from build123d import *

# Parameters (mm, degrees)
F0_W         = 27.2
F0_H         = 4.4
F0_W_2       = 4.4
F0_H_2       = 33.7
F1_DEPTH     = 3
F2_R         = 2.99999
F3_DEPTH     = 2
F4_W         = 4.4
F4_H         = 4.4
F5_DEPTH     = 1
F6_T1_DEPTH  = 16
F6_T4_ANGLE  = 90
F6_T6_ANGLE  = 90
F6_T8_ANGLE  = 90
F6_T10_ANGLE = 90


# Not quite as in the source:
# - a fillet or chamfer that OpenCascade refuses, or shapes differently, is made with other operations: its cross-section is extruded or revolved along the edge and cut away or added
# - a fillet or chamfer is up to 0.001 mm smaller than in the source, because OpenCascade refuses the exact size


with BuildPart() as f1:
    # F0 (on Top) → F1 (new body)
    with BuildSketch(Plane.XY):
        with Locations((0.1669520199, 19.5440534235)):
            Rectangle(F0_W, F0_H)
        with Locations((-15.6330479801, 0.4940534235)):
            Rectangle(F0_W_2, F0_H_2)
        with Locations((-15.6330479801, 19.5440534235)):
            Rectangle(F0_W_2, F0_H)
        with Locations((-15.6330479801, -18.5559465765)):
            Rectangle(F0_W_2, F0_H)
        with Locations((0.1669520199, -18.5559465765)):
            Rectangle(F0_W, F0_H)
        with Locations((15.9669520199, -18.5559465765)):
            Rectangle(F0_W_2, F0_H)
        with Locations((15.9669520199, 0.4940534235)):
            Rectangle(F0_W_2, F0_H_2)
        with Locations((15.9669520199, 19.5440534235)):
            Rectangle(F0_W_2, F0_H)
    extrude(amount=F1_DEPTH)

    # F2 (radius 3 in the source; OpenCascade refuses exactly that, so slightly less here)
    f2_edges = [f1.edges().sort_by_distance(p)[0] for p in [
        (18.166952, 0.494053, 3),
        (0.166952, 21.744053, 3),
        (-17.833048, 0.494053, 3),
        (0.166952, -20.755947, 3),
    ]]
    fillet(f2_edges, radius=F2_R)

    # F0 (on Top) → F3 (join)
    with BuildSketch(Plane.XY):
        with Locations((-15.6330479801, -18.5559465765)):
            Rectangle(F0_W_2, F0_H)
        with Locations((15.9669520199, -18.5559465765)):
            Rectangle(F0_W_2, F0_H)
        with Locations((15.9669520199, 19.5440534235)):
            Rectangle(F0_W_2, F0_H)
        with Locations((-15.6330479801, 19.5440534235)):
            Rectangle(F0_W_2, F0_H)
    extrude(amount=-F3_DEPTH)

    # F4 (on face) → F5 (join)
    with BuildSketch(Plane(origin=(0, 0, -2), x_dir=(1, 0, 0), z_dir=(0, 0, -1))):
        Polygon((-13.4330479801, -21.7440534235), (18.1669520199, -21.7440534235), (18.1669520199, 20.7559465765), (-17.8330479801, 20.7559465765), (-17.8330479801, -17.3440534235), (-13.4330479801, -17.3440534235), align=None)
        with Locations((-15.6330479801, -19.5440534235)):
            Rectangle(F4_W, F4_H)
    extrude(amount=F5_DEPTH)

    # F6: fillet of radius 4 on 4 edges, made by hand

    # F6_s2 → F6_t1 (cut)
    with BuildSketch(Plane.XY.offset(-13)):
        with BuildLine():
            ThreePointArc((18.1669520199, 17.7440534235), (16.9953791447, 20.5724805482), (14.1669520199, 21.7440534235))
            Line((14.1669520199, 21.7440534235), (18.1669520199, 21.7440534235))
            Line((18.1669520199, 21.7440534235), (18.1669520199, 17.7440534235))
        make_face()
        with BuildLine():
            ThreePointArc((18.1669520199, -16.7559465765), (16.9953791447, -19.5843737013), (14.1669520199, -20.7559465765))
            Line((14.1669520199, -20.7559465765), (18.1669520199, -20.7559465765))
            Line((18.1669520199, -20.7559465765), (18.1669520199, -16.7559465765))
        make_face()
        with BuildLine():
            ThreePointArc((-17.8330479801, -16.7559465765), (-16.6614751048, -19.5843737013), (-13.8330479801, -20.7559465765))
            Line((-13.8330479801, -20.7559465765), (-17.8330479801, -20.7559465765))
            Line((-17.8330479801, -20.7559465765), (-17.8330479801, -16.7559465765))
        make_face()
        with BuildLine():
            ThreePointArc((-17.8330479801, 17.7440534235), (-16.6614751048, 20.5724805482), (-13.8330479801, 21.7440534235))
            Line((-13.8330479801, 21.7440534235), (-17.8330479801, 21.7440534235))
            Line((-17.8330479801, 21.7440534235), (-17.8330479801, 17.7440534235))
        make_face()
    extrude(amount=F6_T1_DEPTH, mode=Mode.SUBTRACT)

    # F6_s3 → F6_t4 (revolve, cut)
    with BuildSketch(Plane.YZ.offset(-13.8330479801)):
        with BuildLine():
            ThreePointArc((18.7440634235, 3), (20.8653766959, 2.1213232725), (21.7440534235, 1e-05))
            Line((21.7440534235, 1e-05), (21.7440534235, 3))
            Line((21.7440534235, 3), (18.7440634235, 3))
        make_face()
    revolve(axis=Axis((-13.8330479801, 17.7440534235, 3), (0, 0, 1)), revolution_arc=F6_T4_ANGLE, mode=Mode.SUBTRACT)

    # F6_s5 → F6_t6 (revolve, cut)
    with BuildSketch(Plane.XZ.offset(16.7559465765)):
        with BuildLine():
            ThreePointArc((-14.8330579801, 3), (-16.9543712526, 2.1213232725), (-17.8330479801, 1e-05))
            Line((-17.8330479801, 1e-05), (-17.8330479801, 3))
            Line((-17.8330479801, 3), (-14.8330579801, 3))
        make_face()
    revolve(axis=Axis((-13.8330479801, -16.7559465765, 3), (0, 0, 1)), revolution_arc=F6_T6_ANGLE, mode=Mode.SUBTRACT)

    # F6_s7 → F6_t8 (revolve, cut)
    with BuildSketch(Plane.YZ.offset(14.1669520199)):
        with BuildLine():
            ThreePointArc((-17.7559565765, 3), (-19.877269849, 2.1213232725), (-20.7559465765, 1e-05))
            Line((-20.7559465765, 1e-05), (-20.7559465765, 3))
            Line((-20.7559465765, 3), (-17.7559565765, 3))
        make_face()
    revolve(axis=Axis((14.1669520199, -16.7559465765, 3), (0, 0, 1)), revolution_arc=F6_T8_ANGLE, mode=Mode.SUBTRACT)

    # F6_s9 → F6_t10 (revolve, cut)
    with BuildSketch(Plane.XZ.offset(-17.7440534235)):
        with BuildLine():
            ThreePointArc((15.1669620199, 3), (17.2882752924, 2.1213232725), (18.1669520199, 1e-05))
            Line((18.1669520199, 1e-05), (18.1669520199, 3))
            Line((18.1669520199, 3), (15.1669620199, 3))
        make_face()
    revolve(axis=Axis((14.1669520199, 17.7440534235, 3), (0, 0, 1)), revolution_arc=F6_T10_ANGLE, mode=Mode.SUBTRACT)


solid = f1.part
Build history of the part. All positions in model axes, mm. A direction names the side the tool comes from. Give positions to 0.01 mm unless a question says otherwise; leave off trailing zeros. Loops run counter-clockwise (first coordinate to the right, second up) from the corner with the lowest first, then second, coordinate; pieces in that order, holes last. Notation, with made-up numbers: (13, 20) - (54, 20) arc R27 cw to (54, 53) - close; hole circle Ø9 at (-31, 18). An arc over 180 degrees is marked (long way). Write item = value, one per line. Start each with the question number.
1) Band-saw the part on B-B on z = -0.5. Give the cut face in (x, y).
2) Drop flat-ended pins along their axis: pin 1 Ø1 at (x, z) = (17, -1.5) entering from -Y; pin 2 Ø2 at (y, z) = (19, -1.5) entering from +X; pin 3 Ø2 at (x, z) = (9, 1.5) entering from +Y. Give the stop position or say it passes through.
3) Band-saw the part on A-A on x = -8. Count the separate pieces of the cut face and the enclosed holes in it, plus the area to 3 significant figures.
4) Tool access for faces 1 (the flat face through (-13.433, 0, 1)), 2 (the flat face through (-13.433, 20, -1)), 3 (the flat face through (-16, 17.344, -1)): list every direction of +Z, -Z, +X, -X, +Y, -Y with a clear straight run to the whole face (end or side of a thin tool).
5) Pull direction Y, two halves, no side cores. Call faces 4 (the flat face through (0, 20, 0)), 5 (the cylindrical face through (-16.692, -19.553, -1.521)), 6 (the flat face through (0, 0, -2)): +Y half, -Y half, draft (parallel to the pull), parting line (faces both ways), or undercut.
6) Probe probe 1 along Z at (x, y) = (14, 16); probe 2 along Z at (x, y) = (-8.5, 0.5); probe 3 along X at (y, z) = (-0.5, 2). List the from-to ranges inside material, lowest first. Write a range as from..to.
Final values:
q1.outline = (-17.83, -16.76) arc R4 ccw to (-13.83, -20.76) - (-13.43, -20.76) - (-13.43, -16.36) - (-17.83, -16.36) - close; (-17.83, 17.34) - (-13.43, 17.34) - (-13.43, 21.74) - (-13.83, 21.74) arc R4 ccw to (-17.83, 17.74) - close; (13.77, -20.76) - (14.17, -20.76) arc R4 ccw to (18.17, -16.76) - (18.17, -16.36) - (13.77, -16.36) - close; (13.77, 17.34) - (18.17, 17.34) - (18.17, 17.74) arc R4 ccw to (14.17, 21.74) - (13.77, 21.74) - close
q2.pin_1 = -20.01
q2.pin_2 = 18.16
q2.pin_3 = 21.7
q3.separate_pieces = 3
q3.enclosed_holes = 0
q3.area = 65.0 mm²
q4.face_1 = +Z
q4.face_2 = +Y, -Y
q4.face_3 = +X, -X
q5.face_4 = draft
q5.face_5 = -Y half
q5.face_6 = undercut
q6.probe_1 = -3..-2, 0..3
q6.probe_2 = -3..-2
q6.probe_3 = -17.07..-13.43, 13.77..17.4
